The listing builds one solid part. Answer for the finished solid, in the listing's coordinates (mm). A direction names the side the tool comes from. Coordinates: 2 decimals unless noted, no trailing zeros. Loops run counter-clockwise (first coordinate to the right, second up) from the corner with the lowest first, then second, coordinate; pieces in that order, holes last. Notation, with made-up numbers: (57, 24.5) -> (76, 24.5) arc R7 ccw to (76, 36.5) -> close; hole circle Ø11 at (10.5, -2.75). An arc over 180 degrees is marked (long way). Answer in a Markdown table with one row per item.
```python
from build123d import *

# Parameters (mm, degrees)
SKETCH1_R           = 20.45
SKETCH1_R_2         = 1.65
SKETCH1_R_3         = 1.650080795
BOSS_EXTRUDE1_DEPTH = 4
BOSS_EXTRUDE2_START = -15.91
SKETCH1_4_R         = 1.65
SKETCH1_4_R_2       = 1.650080795
BOSS_EXTRUDE2_DEPTH = 15.91


with BuildPart() as part:
    # Sketch1 → Boss-Extrude1 (new body)
    # profile 1 of 5: a face of its own
    with BuildSketch(Plane.XY):
        Polygon((-13.662202379, -21.5), (13.662202379, -21.5), (13.662202379, -16.5), (16.5, -13.662202379), (21.5, -13.662202379), (21.5, 13.662202379), (16.5, 13.662202379), (13.662202379, 16.5), (13.662202379, 21.5), (-13.662202379, 21.5), (-13.662202379, 16.5), (-16.5, 13.662202379), (-21.5, 13.662202379), (-21.5, -13.662202379), (-16.5, -13.662202379), (-13.662202379, -16.5), align=None)
        Circle(SKETCH1_R, mode=Mode.SUBTRACT)
    # profile 2 of 5: a face of its own
    with BuildSketch(Plane.XY):
        Polygon((13.662202379, -21.5), (19.162202379, -21.5), (21.5, -19.162202379), (21.5, -13.662202379), (16.5, -13.662202379), (13.662202379, -16.5), align=None)
        with Locations((17.621156877, -17.621156877)):
            Circle(SKETCH1_R_2, mode=Mode.SUBTRACT)
    # profile 3 of 5: a face of its own
    with BuildSketch(Plane.XY):
        Polygon((-19.162202379, -21.5), (-13.662202379, -21.5), (-13.662202379, -16.5), (-16.5, -13.662202379), (-21.5, -13.662202379), (-21.5, -19.162202379), align=None)
        with Locations((-17.621156877, -17.621156877)):
            Circle(SKETCH1_R_3, mode=Mode.SUBTRACT)
    # profile 4 of 5: a face of its own
    with BuildSketch(Plane.XY):
        Polygon((-21.5, 19.162202379), (-21.5, 13.662202379), (-16.5, 13.662202379), (-13.662202379, 16.5), (-13.662202379, 21.5), (-19.162202379, 21.5), align=None)
        with Locations((-17.621156877, 17.621156877)):
            Circle(SKETCH1_R_2, mode=Mode.SUBTRACT)
    # profile 5 of 5: a face of its own
    with BuildSketch(Plane.XY):
        Polygon((16.5, 13.662202379), (21.5, 13.662202379), (21.5, 19.162202379), (19.162202379, 21.5), (13.662202379, 21.5), (13.662202379, 16.5), align=None)
        with Locations((17.621156877, 17.621156877)):
            Circle(SKETCH1_R_2, mode=Mode.SUBTRACT)
    extrude(amount=BOSS_EXTRUDE1_DEPTH)

    # Sketch1_4 → Boss-Extrude2 (add)
    # profile 1 of 4: a face of its own
    with BuildSketch(Plane.XY.offset(BOSS_EXTRUDE2_START)):
        Polygon((13.662202379, -21.5), (19.162202379, -21.5), (21.5, -19.162202379), (21.5, -13.662202379), (16.5, -13.662202379), (13.662202379, -16.5), align=None)
        with Locations((17.621156877, -17.621156877)):
            Circle(SKETCH1_4_R, mode=Mode.SUBTRACT)
    # profile 2 of 4: a face of its own
    with BuildSketch(Plane.XY.offset(BOSS_EXTRUDE2_START)):
        Polygon((16.5, 13.662202379), (21.5, 13.662202379), (21.5, 19.162202379), (19.162202379, 21.5), (13.662202379, 21.5), (13.662202379, 16.5), align=None)
        with Locations((17.621156877, 17.621156877)):
            Circle(SKETCH1_4_R, mode=Mode.SUBTRACT)
    # profile 3 of 4: a face of its own
    with BuildSketch(Plane.XY.offset(BOSS_EXTRUDE2_START)):
        Polygon((-21.5, 19.162202379), (-21.5, 13.662202379), (-16.5, 13.662202379), (-13.662202379, 16.5), (-13.662202379, 21.5), (-19.162202379, 21.5), align=None)
        with Locations((-17.621156877, 17.621156877)):
            Circle(SKETCH1_4_R, mode=Mode.SUBTRACT)
    # profile 4 of 4: a face of its own
    with BuildSketch(Plane.XY.offset(BOSS_EXTRUDE2_START)):
        Polygon((-19.162202379, -21.5), (-13.662202379, -21.5), (-13.662202379, -16.5), (-16.5, -13.662202379), (-21.5, -13.662202379), (-21.5, -19.162202379), align=None)
        with Locations((-17.621156877, -17.621156877)):
            Circle(SKETCH1_4_R_2, mode=Mode.SUBTRACT)
    extrude(amount=BOSS_EXTRUDE2_DEPTH)


solid = part.part
```
Item 1: A cutting plane is placed at C-C, the plane z = -3. Determine the outline of the cut face in (x, y).
Findings below:
| item | result |
|---|---|
| outline | (-21.5, -19.16) -> (-19.16, -21.5) -> (-13.66, -21.5) -> (-13.66, -16.5) -> (-16.5, -13.66) -> (-21.5, -13.66) -> close; (-21.5, 13.66) -> (-16.5, 13.66) -> (-13.66, 16.5) -> (-13.66, 21.5) -> (-19.16, 21.5) -> (-21.5, 19.16) -> close; (13.66, -21.5) -> (19.16, -21.5) -> (21.5, -19.16) -> (21.5, -13.66) -> (16.5, -13.66) -> (13.66, -16.5) -> close; (13.66, 16.5) -> (16.5, 13.66) -> (21.5, 13.66) -> (21.5, 19.16) -> (19.16, 21.5) -> (13.66, 21.5) -> close; hole circle Ø3.3 at (-17.62, -17.62); hole circle Ø3.3 at (-17.62, 17.62); hole circle Ø3.3 at (17.62, -17.62); hole circle Ø3.3 at (17.62, 17.62) |
Item 2: A cutting plane is placed at D-D, the plane z = 2.5. Determine the outline of the cut face in (x, y).
Findings below:
| item | result |
|---|---|
| outline | (-21.5, -19.16) -> (-19.16, -21.5) -> (19.16, -21.5) -> (21.5, -19.16) -> (21.5, 19.16) -> (19.16, 21.5) -> (-19.16, 21.5) -> (-21.5, 19.16) -> close; hole circle Ø40.9 at (0, 0); hole circle Ø3.3 at (-17.62, -17.62); hole circle Ø3.3 at (-17.62, 17.62); hole circle Ø3.3 at (17.62, -17.62); hole circle Ø3.3 at (17.62, 17.62) |
Item 3: Find the intervals of material crossed by probe 1 along Y at (x, z) = (0, 1.55); probe 2 along Y at (x, z) = (15, -14); probe 3 along Z at (x, y) = (-19.5, -11), in increasing order.
Findings below:
| item | result |
|---|---|
| probe 1 | y = -21.5 to -20.45, 20.45 to 21.5 |
| probe 2 | y = -21.5 to -15.16, 15.16 to 21.5 |
| probe 3 | z = 0 to 4 |
Item 4: A tool of negligible diameter and unlimited length cuts with its end or side. For faces 1 (the face through (-15.06, -15.1, -8.07)), 2 (the face through (13.662, 19, -8)), 3 (the face through (19, -13.662, -8)), from which of +Z, -Z, +X, -X, +Y, -Y can it reach the whole face along a straight path? Write none if from no direction.
Findings below:
| item | result |
|---|---|
| face 1 | -Z |
| face 2 | -Z, +Y, -Y |
| face 3 | -Z, +X, -X |
Item 5: A cutting plane is placed at A-A, the plane x = 0. Determine the outline of the cut face in (y, z), plus the area to 3 significant figures.
Findings below:
| item | result |
|---|---|
| outline | (-21.5, 0) -> (-20.45, 0) -> (-20.45, 4) -> (-21.5, 4) -> close; (20.45, 0) -> (21.5, 0) -> (21.5, 4) -> (20.45, 4) -> close |
| area | 8.40 mm2 |
Item 6: Determine the mould class of faces 4 (the face through (-13, 16, 0)), 5 (the face through (-13.662, -19, -8)), 6 (the face through (0, -21.5, 1)) for opening direction Y: +Y half, -Y half, draft (parallel to the pull), parting line (faces both ways), or undercut.
Findings below:
| item | result |
|---|---|
| face 4 | undercut |
| face 5 | draft |
| face 6 | -Y half |
Item 7: A flat-ended cylindrical pin translates along its axis: pin 1 Ø3 at (x, y) = (17.62, -17.62) entering from -Z. Find the tip coordinate at first contact, or state that the pin passes through.
Findings below:
| item | result |
|---|---|
| pin 1 | passes through |
